Could you check a few things on this model? Use its own coordinates, in mm. Coordinates: 2 decimals unless noted, no trailing zeros. Loops run counter-clockwise (first coordinate to the right, second up) from the corner with the lowest first, then second, coordinate; pieces in that order, holes last. Notation, with made-up numbers: (13.25, 8) -> (56.25, 8) arc R17 cw to (56.25, 25) -> close; hole circle Ø9 at (-26.5, 12.25). An arc over 180 degrees is marked (long way). One line per question, with ' | ' between items.
from build123d import *

# Parameters (mm, degrees)
SKETCH1_R             = 57.15
BOSS_EXTRUDE1_DEPTH   = 2.54
F_8_32_TAPPED_HOLE1_D = 3.4544
CIRPATTERN2_COUNT     = 4


with BuildPart() as part:
    # Sketch1 → Boss-Extrude1 (new body)
    with BuildSketch(Plane(origin=(0, 0, 0), x_dir=(1, 0, 0), z_dir=(0, 1, 0))):
        with Locations(Location((0, 0, 0), (0, 0, 270))):
            Circle(SKETCH1_R)
    extrude(amount=BOSS_EXTRUDE1_DEPTH)

    # #8-32 Tapped Hole1 (through all)
    with Locations(Plane(origin=(0, 2.54, 0), x_dir=(1, 0, 0), z_dir=(0, 1, 0))):
        with Locations((-53.34, 0)):
            f_8_32_tapped_hole1 = Hole(F_8_32_TAPPED_HOLE1_D / 2)

    # CirPattern2: #8-32 Tapped Hole1 ×4 about axis
    cirpattern2_axis = Axis((0, 0, 0), (0, 1, 0))
    for i in range(1, CIRPATTERN2_COUNT):
        add(f_8_32_tapped_hole1.rotate(cirpattern2_axis, i * 360 / CIRPATTERN2_COUNT), mode=Mode.SUBTRACT)


solid = part.part
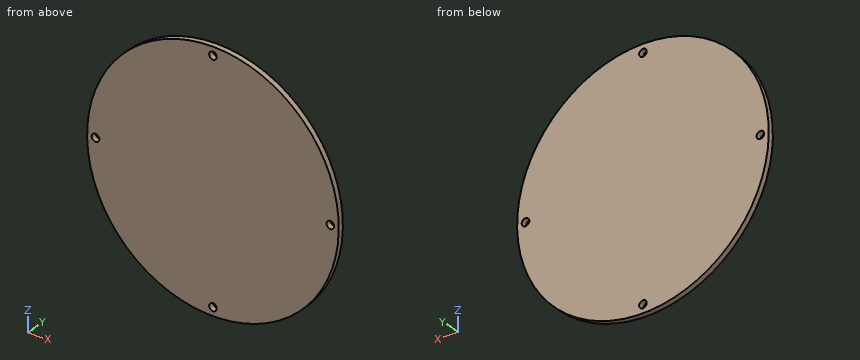
1) If we section it at C-C on y = 1.7: Please give me the cut outline in (x, z).
Data:
outline: circle Ø114.3 at (0, 0); hole circle Ø3.45 at (-53.34, 0); hole circle Ø3.45 at (0, -53.34); hole circle Ø3.45 at (0, 53.34); hole circle Ø3.45 at (53.34, 0)
2) I need wall thicknesses on line 1 along X through (y, z) = (1.8, 1); line 2 along X through (y, z) = (1.4, -52); line 3 along X through (y, z) = (1.2, 16). Which ranges of each line are inside material? Lowest first, please. Write a range as from..to.
Data:
line 1: -57.14..-54.75, -51.93..51.93, 54.75..57.14 | line 2: -23.71..-1.09, 1.09..23.71 | line 3: -54.86..54.86
3) If we section it at B-B on z = 0: Please give me the cut outline in (x, y), and give its area (3 significant figures).
Data:
outline: (-57.15, 0) -> (-55.07, 0) -> (-55.07, 2.54) -> (-57.15, 2.54) -> close; (-51.61, 0) -> (51.61, 0) -> (51.61, 2.54) -> (-51.61, 2.54) -> close; (55.07, 0) -> (57.15, 0) -> (57.15, 2.54) -> (55.07, 2.54) -> close | area: 273 mm²
4) If we section it at D-D on z = 53.34: Please give me the cut outline in (x, y).
Data:
outline: (-20.52, 0) -> (-1.73, 0) -> (-1.73, 2.54) -> (-20.52, 2.54) -> close; (1.73, 0) -> (20.52, 0) -> (20.52, 2.54) -> (1.73, 2.54) -> close
5) If we section it at A-A on x = 0: Please give me the cut outline in (y, z), and give its area (3 significant figures).
Data:
outline: (0, -57.15) -> (2.54, -57.15) -> (2.54, -55.07) -> (0, -55.07) -> close; (0, -51.61) -> (2.54, -51.61) -> (2.54, 51.61) -> (0, 51.61) -> close; (0, 55.07) -> (2.54, 55.07) -> (2.54, 57.15) -> (0, 57.15) -> close | area: 273 mm²
